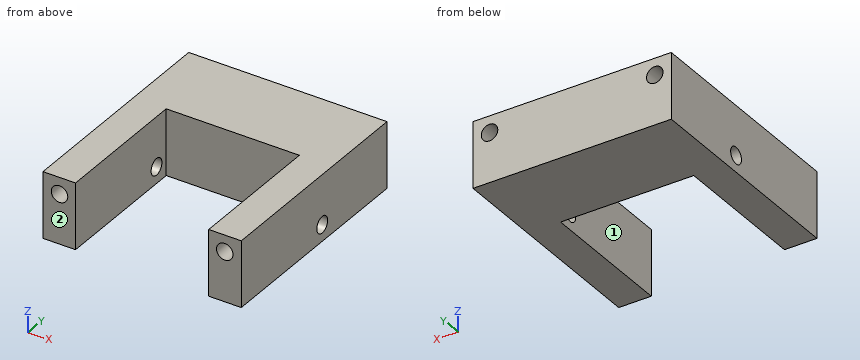
from build123d import *

# Parameters (mm, degrees)
BOSS_EXTRUDE1_DEPTH = 20
SKETCH3_R           = 2.5
CUT_EXTRUDE1_DEPTH  = 68.5
SKETCH4_R           = 2.5
CUT_EXTRUDE2_DEPTH  = 61


with BuildPart() as part:
    # Sketch1 → Boss-Extrude1 (new body)
    with BuildSketch(Plane.XY):
        Polygon((50.15, 0), (60, 0), (60, 67.5), (0, 67.5), (0, 0), (9.85, 0), (9.85, 42), (50.15, 42), align=None)
    extrude(amount=BOSS_EXTRUDE1_DEPTH)

    # Sketch3 → Cut-Extrude1 (cut, through all)
    with BuildSketch(Plane.XZ):
        with Locations((5, 15)):
            Circle(SKETCH3_R)
        with Locations((55, 15)):
            Circle(SKETCH3_R)
    extrude(amount=-CUT_EXTRUDE1_DEPTH, mode=Mode.SUBTRACT)

    # Sketch4 → Cut-Extrude2 (cut, through all)
    with BuildSketch(Plane.ZY):
        with Locations((5, 37.5)):
            Circle(SKETCH4_R)
    extrude(amount=-CUT_EXTRUDE2_DEPTH, mode=Mode.SUBTRACT)


solid = part.part
Verification items for the finished model (mm, model axes). Face numbers are marked on the shaded views. A direction names the side the tool comes from. Give positions to 0.01 mm unless a question says otherwise; leave off trailing zeros. Write each loop counter-clockwise with the first axis right and the second up, starting at its lowest first coordinate (ties: lowest second). Pieces come first, ordered by that corner, then holes.
(1) Gauge pin test, flat ends, axial feed: pin 1 (12 mm diameter, centred on x = 14, y = 41, fed in from -Z); pin 2 (6 mm diameter, centred on x = 23, z = 10.5, fed in from -Y); pin 3 (4 mm diameter, centred on y = 37.5, z = 5, fed in from +X). Record the tip position at first contact, or that the pin passes through.
(2) Cross-section at A-A (x = 5). Enter the section's corners in (y, z).
(3) Access from +Z, -Z, +X, -X, +Y, -Y to the whole of each face (thin tool, end or side, straight path). Record for the marked faces 1 and 2.
(4) Cross-section at B-B (y = 7). Enter the section's corners in (x, z), plus the area to 3 significant figures.
(5) Cross-section at D-D (y = 60). Enter the section's corners in (x, z).
(6) Material ranges on line 1 (X direction, y = 29, z = 1.5); line 2 (X direction, y = 27, z = 14.5); line 3 (X direction, y = 24, z = 16.5), recorded low to high.
(7) Cross-section at C-C (z = 6.5). Enter the section's corners in (x, y), plus the area to 3 significant figures.
Worked out:
1. pin 1: stops at z = 0
1. pin 2: stops at y = 42
1. pin 3: passes through
2. outline: (0, 0) - (67.5, 0) - (67.5, 12.5) - (0, 12.5) - close; (0, 17.5) - (67.5, 17.5) - (67.5, 20) - (0, 20) - close; hole circle Ø5 at (37.5, 5)
3. face 1: +Z, -Z, -Y
3. face 2: +Z, -Z, +X, -X, -Y
4. outline: (0, 0) - (9.85, 0) - (9.85, 20) - (0, 20) - close; (50.15, 0) - (60, 0) - (60, 20) - (50.15, 20) - close; hole circle Ø5 at (5, 15); hole circle Ø5 at (55, 15)
4. area: 355 mm2
5. outline: (0, 0) - (60, 0) - (60, 20) - (0, 20) - close; hole circle Ø5 at (5, 15); hole circle Ø5 at (55, 15)
6. line 1: x = 0 to 9.85, 50.15 to 60
6. line 2: x = 0 to 2.55, 7.45 to 9.85, 50.15 to 52.55, 57.45 to 60
6. line 3: x = 0 to 3, 7 to 9.85, 50.15 to 53, 57 to 60
7. outline: (0, 0) - (9.85, 0) - (9.85, 35.5) - (0, 35.5) - close; (0, 39.5) - (9.85, 39.5) - (9.85, 42) - (50.15, 42) - (50.15, 39.5) - (60, 39.5) - (60, 67.5) - (0, 67.5) - close; (50.15, 0) - (60, 0) - (60, 35.5) - (50.15, 35.5) - close
7. area: 2,280 mm2
